Source: CAD feature listing. Evaluate the final solid. Frame: model axes, mm. Give positions to 0.01 mm unless a question says otherwise; leave off trailing zeros. Loops run counter-clockwise (first coordinate to the right, second up) from the corner with the lowest first, then second, coordinate; pieces in that order, holes last. Notation, with made-up numbers: M 8,85 L 59,85 A35 ccw 59,117 Z; hole C 23.5,16 d2. An arc over 180 degrees is marked long. Answer in a Markdown table with one row per item.
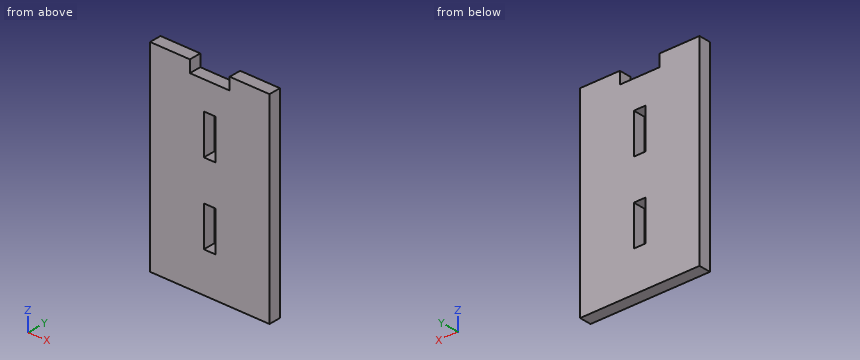
```python
from build123d import *

# Parameters (mm, degrees)
CROQUIS1_W              = 3
CROQUIS1_H              = 10
SALIENTE_EXTRUIR1_DEPTH = 3


with BuildPart() as part:
    # Croquis1 → Saliente-Extruir1 (new body)
    with BuildSketch(Plane(origin=(0, 0, 0), x_dir=(1, 0, 0), z_dir=(0, 1, 0))):
        Polygon((25, 0), (35, 0), (35, 50), (5, 50), (5, 0), (15, 0), (15, 3), (25, 3), align=None)
        with Locations((20, 15)):
            Rectangle(CROQUIS1_W, CROQUIS1_H, mode=Mode.SUBTRACT)
        with Locations((20, 35)):
            Rectangle(CROQUIS1_W, CROQUIS1_H, mode=Mode.SUBTRACT)
    extrude(amount=SALIENTE_EXTRUIR1_DEPTH)


solid = part.part
```
Q1. Section query D-D (x = 24). Output: boundary loops of the cut face in (y, z), plus the area to 3 significant figures.
Values follow:
| item | result |
|---|---|
| outline | M 0,-50 L 3,-50 L 3,-3 L 0,-3 Z |
| area | 141 mm^2 |
Q2. Section query C-C (y = 2.5). Output: boundary loops of the cut face in (x, z).
Values follow:
| item | result |
|---|---|
| outline | M 5,-50 L 35,-50 L 35,0 L 25,0 L 25,-3 L 15,-3 L 15,0 L 5,0 Z; hole M 18.5,-40 L 21.5,-40 L 21.5,-30 L 18.5,-30 Z; hole M 18.5,-20 L 21.5,-20 L 21.5,-10 L 18.5,-10 Z |
Q3. Contact query for a flat-ended pin moving along its axis: pin 1 Ø0.9 at (x, y) = (20, 1) entering from +Z. Output: stop coordinate, or through.
Values follow:
| item | result |
|---|---|
| pin 1 | z = -3 |
Q4. Ray query, probe 1 along Z at (x, y) = (19.75, 2.85); probe 2 along X at (y, z) = (2.45, -32.5); probe 3 along Z at (x, y) = (15.5, 1.3). Return the intervals inside material, ascending. Write a range as from..to.
Values follow:
| item | result |
|---|---|
| probe 1 | -50..-40, -30..-20, -10..-3 |
| probe 2 | 5..18.5, 21.5..35 |
| probe 3 | -50..-3 |
Q5. Section query B-B (x = 19.25). Output: boundary loops of the cut face in (y, z).
Values follow:
| item | result |
|---|---|
| outline | M 0,-50 L 3,-50 L 3,-40 L 0,-40 Z; M 0,-30 L 3,-30 L 3,-20 L 0,-20 Z; M 0,-10 L 3,-10 L 3,-3 L 0,-3 Z |
Q6. Section query A-A (z = -17.5). Output: boundary loops of the cut face in (x, y).
Values follow:
| item | result |
|---|---|
| outline | M 5,0 L 18.5,0 L 18.5,3 L 5,3 Z; M 21.5,0 L 35,0 L 35,3 L 21.5,3 Z |
